```python
from build123d import *

# Parameters (mm, degrees)
SKE1_R      = 6.5
BASE1_DEPTH = 8
BODYSKE_W   = 20
BODYSKE_H   = 4
HEX_2_DEPTH = 4


with BuildPart() as part:
    # Ske1 → Base1 (new body)
    with BuildSketch(Plane.XY):
        Circle(SKE1_R)
    extrude(amount=BASE1_DEPTH)

    # BodySke → BaseBody (revolve)
    with BuildSketch(Plane(origin=(0, 0, 0), x_dir=(0, 0, -1), z_dir=(1, 0, 0)), mode=Mode.PRIVATE) as basebody_sk:
        with Locations((2, 2)):
            Rectangle(BODYSKE_W, BODYSKE_H)
    revolve(basebody_sk.sketch.rotate(Axis((0, 0, 1.385793675), (0, 0, -1)), 90), axis=Axis((0, 0, 1.385793675), (0, 0, -1)))

    # Ske8 → Hex 2 (cut)
    with BuildSketch(Plane.XY.offset(8)):
        Polygon((0, 3.464101615), (-3, 1.732050808), (-3, -1.732050808), (0, -3.464101615), (3, -1.732050808), (3, 1.732050808), align=None)
    extrude(amount=-HEX_2_DEPTH, mode=Mode.SUBTRACT)

    # Chamfer 2 cone 1 section (through the dimple's axis) → Chamfer 2 (revolve, cut)
    with BuildSketch(Plane(origin=(0, 0, 8), x_dir=(0, -1, 0), z_dir=(1, 0, 0))):
        Polygon((0, 0), (3.6, 0), (0, 2.078460969), align=None)
    revolve(axis=Axis((0, 0, 8), (0, 0, -1)), mode=Mode.SUBTRACT)


solid = part.part
```
CAD build for the part. Positions are in the model's coordinates, mm. A direction names the side the tool comes from. Round coordinates to 2 decimals unless told otherwise and drop trailing zeros. Order: outer loops, then holes, each group sorted by start corner. A loop starts at its lowest first (then second) coordinate and runs counter-clockwise, first axis right, second up.
Q1. Slice it at D-D (y = 5.75). Write the cut outline in (x, z), and give its area (3 significant figures).
Q2. Which spindle directions (+Z, -Z, +X, -X, +Y, -Y) get a long thin tool onto all of the face, cutting with end or side? Do faces 1 (the flat face through (3, 3, 0)), 2 (the flat face through (0, 0, -12)), 3 (the flat face through (-1.5, 2.6, 6)). Say none if no direction does.
Q3. Wall check: L1, parallel to Z at x = 2.75, y = -1.75; L2, parallel to Z at x = 5, y = -2.25; L3, parallel to X at y = 2, z = 6. Give the ranges that are in metal, low to high.
Q4. Slice it at A-A (z = 6.75). Write the cut outline in (x, y).
Q5. Two-plate mould, pull along Y, no slides. Class faces 4 (the cylindrical face through (-5.158, -3.955, 3.944)), 5 (the flat face through (3, 0, 6)), 6 (the flat face through (-3, 3, 8)): pulls with the +Y half, pulls with the -Y half, needs draft (parallel to the pull), parting line crosses it, or undercut.
Q6. Drop flat-ended pins along their axis: pin 1 (6 mm diameter, centred on x = -4.5, z = 6, fed in from -Y); pin 2 (4 mm diameter, centred on x = 2.5, y = -2, fed in from +Z); pin 3 (1.8 mm diameter, centred on x = -1.5, y = 1, fed in from +Z); pin 4 (6 mm diameter, centred on y = -1, z = -8, fed in from -X). Give the stop position or say it passes through.
Q7. Slice it at B-B (y = 0). Write the cut outline in (x, z).
Q8. Slice it at C-C (z = -3.75). Write the cut outline in (x, y).
Results below:
1. outline: (-3.03, 0) - (3.03, 0) - (3.03, 8) - (-3.03, 8) - close
1. area: 48.5 mm2
2. face 1: -Z
2. face 2: -Z, +X, -X, +Y, -Y
2. face 3: +Z
3. L1: z = -12 to 4
3. L2: z = 0 to 8
3. L3: x = -6.18 to -2.54, 2.54 to 6.18
4. outline: circle Ø13 at (0, 0); hole (-3, -1.73) - (0, -3.46) - (3, -1.73) - (3, 1.73) - (0, 3.46) - (-3, 1.73) - close
5. face 4: parting line crosses it
5. face 5: undercut
5. face 6: needs draft
6. pin 1: stops at y = -6.32
6. pin 2: stops at z = 8
6. pin 3: stops at z = 4
6. pin 4: stops at x = -4
7. outline: (-6.5, 0) - (-4, 0) - (-4, -12) - (4, -12) - (4, 0) - (6.5, 0) - (6.5, 8) - (3.6, 8) - (3, 7.65) - (3, 4) - (-3, 4) - (-3, 7.65) - (-3.6, 8) - (-6.5, 8) - close
8. outline: circle Ø8 at (0, 0)
